Could you check a few things on this drawing? It's one solid part, dimensions in mm from its lowest x, y, z. Coordinates: 2 decimals unless noted, no trailing zeros. Write each loop counter-clockwise with the first axis right and the second up, starting at its lowest first coordinate (ties: lowest second). Pieces come first, ordered by that corner, then holes.
Item 1: I want a section at B-B (y = 370). Please give me the cut outline in (x, z), and give its area (3 significant figures).
Item 2: I'm going to push flat-ended pins straight in: P1, Ø6.5, axis at y = 18, z = 18, coming from the -X side; P2, Ø3, axis at x = 4.5, z = 4, coming from the -Y side. Where does each tip first touch, or does it pass through?
Item 3: I want a section at A-A (x = 2). Please give me the cut outline in (y, z).
Item 4: Please list where these lines run through material, in increasing order: line 1 (Y direction, x = 2.25, z = 18); line 2 (Y direction, x = 0.7, z = 18.5); line 3 (Z direction, x = 2.4, y = 18).
Item 5: I want a section at C-C (z = 4.5). Please give me the cut outline in (x, y).
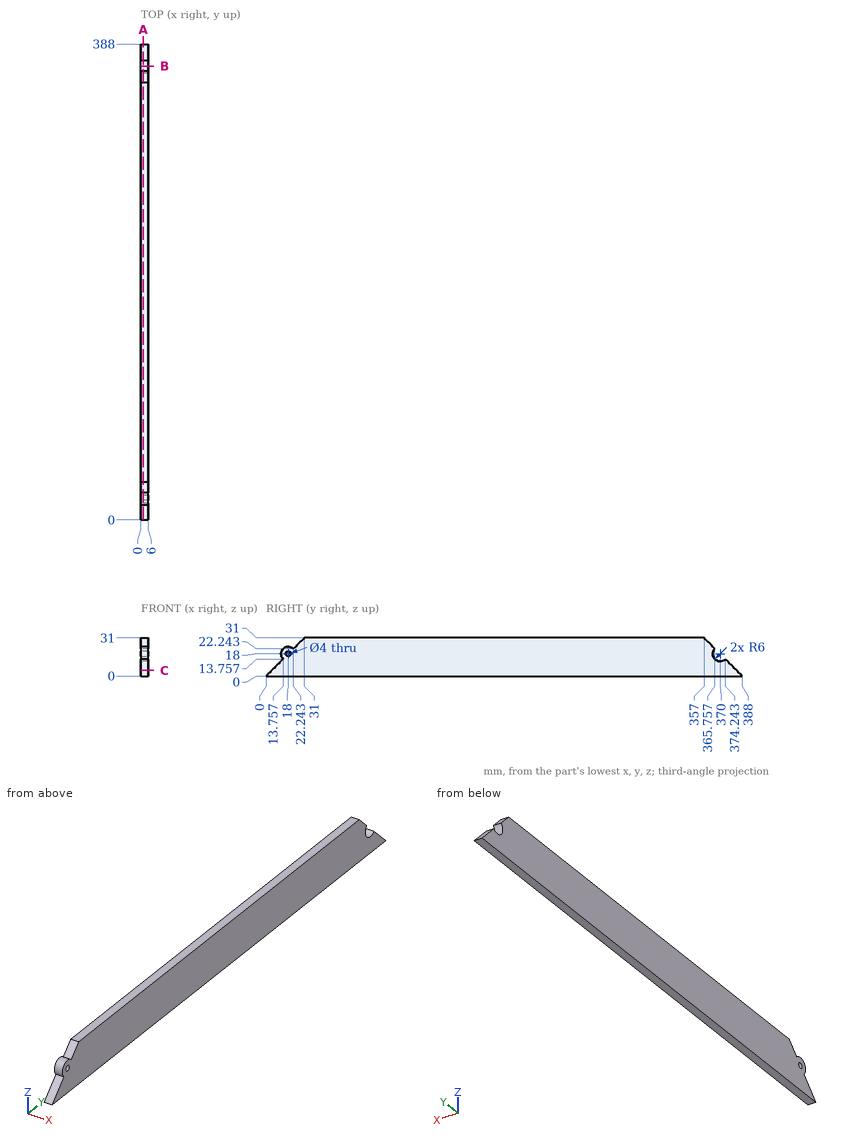
Answer:
1. outline: (0, 0) - (6, 0) - (6, 12) - (0, 12) - close
1. area: 72.0 mm2
2. P1: stops at x = 0
2. P2: stops at y = 2.5
3. outline: (0, 0) - (388, 0) - (374.24, 13.76) arc R6 cw to (365.76, 22.24) - (357, 31) - (31, 31) - (22.24, 22.24) arc R6 ccw to (13.76, 13.76) - close; hole circle Ø4 at (18, 18)
4. line 1: y = 12 to 16, 20 to 364
4. line 2: y = 12.02 to 16.06, 19.94 to 364.02
4. line 3: z = 0 to 16, 20 to 24
5. outline: (0, 4.5) - (6, 4.5) - (6, 383.5) - (0, 383.5) - close
